from build123d import *

# Parameters (mm, degrees)
SKETCH_1_W            = 78
SKETCH_1_H            = 51
EXTRUDE_1_DEPTH       = 28
HOLE_WIZARD_M31_D     = 2.5
HOLE_WIZARD_M31_DEPTH = 5.5
HOLE_WIZARD_M31_TIP   = 0.751075774
HOLE_WIZARD_M32_D     = 2.5
HOLE_WIZARD_M32_DEPTH = 5.5
HOLE_WIZARD_M32_TIP   = 0.751075774
SKETCH_6_W            = 36.55514342
SKETCH_6_H            = 9.362324501
EXTRUDE_2_DEPTH       = 14


with BuildPart() as part:
    # Эскиз1 → Бобышка-Вытянуть1 (new body)
    with BuildSketch(Plane(origin=(0, 0, 0), x_dir=(1, 0, 0), z_dir=(0, 1, 0))):
        Rectangle(SKETCH_1_W, SKETCH_1_H)
    extrude(amount=EXTRUDE_1_DEPTH)

    # Отверстие обработанное метчиком M31
    with Locations(Plane.XY.offset(25.5)):
        with Locations((36.25, 14), (-30.25, 14)):
            Hole(HOLE_WIZARD_M31_D / 2, depth=HOLE_WIZARD_M31_DEPTH)
            with Locations((0, 0, -(HOLE_WIZARD_M31_DEPTH + HOLE_WIZARD_M31_TIP / 2))):  # 118° drill point
                Cone(0, HOLE_WIZARD_M31_D / 2, HOLE_WIZARD_M31_TIP, mode=Mode.SUBTRACT)

    # Отверстие обработанное метчиком M32
    with Locations(Plane(origin=(0, 0, 0), x_dir=(-1, 0, 0), z_dir=(0, -1, 0))):
        with Locations((-28, -0.1), (27, -0.1)):
            Hole(HOLE_WIZARD_M32_D / 2, depth=HOLE_WIZARD_M32_DEPTH)
            with Locations((0, 0, -(HOLE_WIZARD_M32_DEPTH + HOLE_WIZARD_M32_TIP / 2))):  # 118° drill point
                Cone(0, HOLE_WIZARD_M32_D / 2, HOLE_WIZARD_M32_TIP, mode=Mode.SUBTRACT)

    # Эскиз6 → Бобышка-Вытянуть2 (add)
    with BuildSketch(Plane.ZY.offset(39)):
        with Locations((-2.393178454, 8.082800526)):
            Rectangle(SKETCH_6_W, SKETCH_6_H)
    extrude(amount=EXTRUDE_2_DEPTH)


solid = part.part
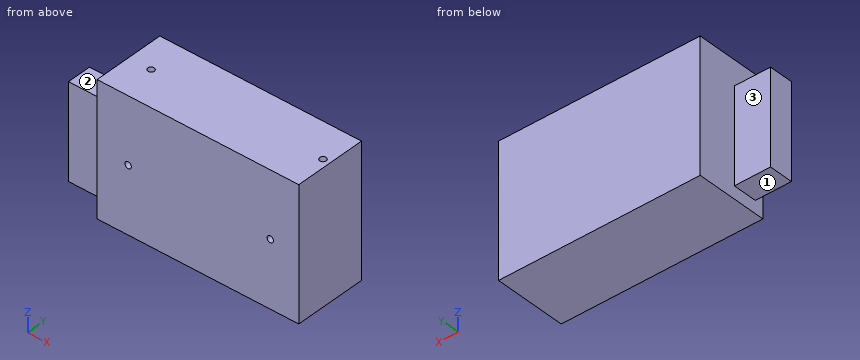
Build history of the part. All positions in model axes, mm. Face numbers are marked on the shaded views. A direction names the side the tool comes from. Round coordinates to 2 decimals unless told otherwise and drop trailing zeros. Write each loop counter-clockwise with the first axis right and the second up, starting at its lowest first coordinate (ties: lowest second). Pieces come first, ordered by that corner, then holes. Notation, with made-up numbers: M 88.5,20.25 L 128.5,20.25 A20 cw 128.5,53.25 Z; hole C -38,33 d7. An arc over 180 degrees is marked long. Use CSV: the item, a comma, the result in double quotes.
1. Saw through at A-A (z = -14.5). Give the cut face in (x, y).
Reply:
outline,"M -53,3.4 L -39,3.4 L -39,0 L 39,0 L 39,28 L -39,28 L -39,12.76 L -53,12.76 Z"
2. Saw through at B-B (y = 7.5). Give the cut face in (x, z), plus the area to 3 significant figures.
Reply:
outline,"M -53,-20.67 L -39,-20.67 L -39,-25.5 L 39,-25.5 L 39,25.5 L -39,25.5 L -39,15.88 L -53,15.88 Z"
area,"4,490 mm²"
3. Saw through at C-C (y = 23). Give the cut face in (x, z), plus the area to 3 significant figures.
Reply:
outline,"M -39,-25.5 L 39,-25.5 L 39,25.5 L -39,25.5 Z"
area,"3,980 mm²"
4. Wall check: probe 1 along X at (y, z) = (14, 23.85); probe 2 along Y at (x, z) = (36.25, 22.75); probe 3 along Z at (x, y) = (28, 3.6). Give the ranges that are in metal, low to high. Write a range as from..to.
Reply:
probe 1,"x = -39..-31.5, -29..35, 37.5..39"
probe 2,"y = 0..12.75, 15.25..28"
probe 3,"z = -25.5..-1.15, 1.35..25.5"
5. Tool access for the marked faces 1, 2 and 3: list every direction of +Z, -Z, +X, -X, +Y, -Y with a clear straight run to the whole face (end or side of a thin tool).
Reply:
face 1,"-Z, -X, +Y, -Y"
face 2,"+Z, -X, +Y, -Y"
face 3,"+Z, -Z, -X, +Y"
6. Flat gauge pins, fed straight in: pin 1 (2 mm diameter, centred on x = 28, z = 0.1, fed in from -Y); pin 2 (5 mm diameter, centred on y = 18.5, z = -14, fed in from -X); pin 3 (5 mm diameter, centred on x = -42.5, y = 13, fed in from -Z). Where does each tip first touch, or does it go through?
Reply:
pin 1,"stops at y = 5.65"
pin 2,"stops at x = -39"
pin 3,"stops at z = -20.67"
